Geometry check sheet. Reference: the model listing, model coordinates, mm. A direction names the side the tool comes from. Round coordinates to 2 decimals unless told otherwise and drop trailing zeros. Write each loop counter-clockwise with the first axis right and the second up, starting at its lowest first coordinate (ties: lowest second). Pieces come first, ordered by that corner, then holes. Notation, with made-up numbers: (-15, 0.5) - (-3, 0.5) arc R34 ccw to (-3, 35.5) - close; hole circle Ø7 at (15.5, 75). An arc over 180 degrees is marked (long way). Return JSON: item names as keys, results as strings. Group by question number.
from build123d import *

# Parameters (mm, degrees)
F1_DEPTH = 57.15
F2_R     = 3.175
F3_DEPTH = 50.801
F4_R     = 6.35
F5_DEPTH = 2.54
F6_R     = 2
F7_DEPTH = 50.801
F8_R     = 1.5875
F9_DEPTH = 12.7


with BuildPart() as f1:
    # F0 (on Front) → F1 (new body)
    with BuildSketch(Plane.XZ):
        Polygon((-25.4, 0), (0, 0), (25.4, 0), (25.4, 31.75), (18.796, 31.75), (18.796, 4.318), (0, 4.318), (-18.796, 4.318), (-18.796, 31.75), (-25.4, 31.75), align=None)
    extrude(amount=F1_DEPTH)

    # F2 (on face) → F3 (cut, through all)
    with BuildSketch(Plane(origin=(-25.4, 0, 0), x_dir=(0, -1, 0), z_dir=(-1, 0, 0))):
        with Locations((12.7, 12.7)):
            Circle(F2_R)
    extrude(amount=-F3_DEPTH, mode=Mode.SUBTRACT)

    # F4 (on face) → F5 (cut)
    with BuildSketch(Plane.XY.offset(4.318)):
        with Locations((0, -44.45)):
            Circle(F4_R)
    extrude(amount=-F5_DEPTH, mode=Mode.SUBTRACT)

    # F6 (on face) → F7 (cut, through all)
    with BuildSketch(Plane(origin=(-25.4, 0, 0), x_dir=(0, -1, 0), z_dir=(-1, 0, 0))):
        with Locations((38.1, 24.13)):
            Circle(F6_R)
        with Locations((47.6, 24.13)):
            Circle(F6_R)
    extrude(amount=-F7_DEPTH, mode=Mode.SUBTRACT)

    # F8 (on face) → F9 (cut)
    with BuildSketch(Plane.XY.offset(31.75)):
        with Locations((-22.098, -3.175)):
            Circle(F8_R)
        with Locations((-22.098, -22.225)):
            Circle(F8_R)
        with Locations((22.098, -3.175)):
            Circle(F8_R)
        with Locations((22.098, -22.225)):
            Circle(F8_R)
    extrude(amount=-F9_DEPTH, mode=Mode.SUBTRACT)


solid = f1.part
1. Material ranges on line 1 along X through (y, z) = (-22, 26.5); line 2 along X through (y, z) = (-55, 18); line 3 along Y through (x, z) = (-22, 24), recorded low to high.
2. Section check D-D (z = 24.13). State how many separate pieces and enclosed holes the cut face has, and give its area (3 significant figures).
3. Mould release check, pull along Y, two halves, no side actions. Record for faces 1 (the face through (0, -57.15, 4)), 2 (the face through (-22, -28, 31.75)), 3 (the face through (-22, -3, 19.05)): pulls with the +Y half, pulls with the -Y half, needs draft (parallel to the pull), parting line crosses it, or undercut.
4. Section check C-C (x = 0). Enter the section's corners in (y, z).
5. Section check A-A (y = -12.7). Enter the section's corners in (x, z) (3 decimals), and give its area (3 significant figures).
6. Section check B-B (z = 8). Enter the section's corners in (x, y).
7. Depth check by flat-ended pin: pin 1 Ø14 at (x, y) = (0, -45) entering from +Z; pin 2 Ø3.5 at (x, y) = (21.5, -3) entering from +Z; pin 3 Ø3 at (x, y) = (-22.098, -22.225) entering from +Z. Enter the tip coordinate at first touch or a pass-through.
8. Tool access check on faces 4 (the face through (22, -22, 19.05)), 5 (the face through (25.4, -28, 16)), 6 (the face through (0, -28, 4.318)). Record the directions out of +Z, -Z, +X, -X, +Y, -Y that give a thin tool (end or side, any length) a straight path to the whole face; none if there is none.
Result sheet:
{
 "1": {"line 1": "x = -25.4 to -23.67, -20.53 to -18.8, 18.8 to 20.53, 23.67 to 25.4", "line 2": "x = -25.4 to -18.8, 18.8 to 25.4", "line 3": "y = -57.15 to -49.6, -45.6 to -40.1, -36.1 to -23.81, -20.64 to -4.76, -1.59 to 0"},
 "2": {"separate pieces": "6", "enclosed holes": "4", "area": "618 mm²"},
 "3": {"face 1": "pulls with the -Y half", "face 2": "needs draft", "face 3": "undercut"},
 "4": {"outline": "(-57.15, 0) - (0, 0) - (0, 4.32) - (-38.1, 4.32) - (-38.1, 1.78) - (-50.8, 1.78) - (-50.8, 4.32) - (-57.15, 4.32) - close"},
 "5": {"outline": "(-25.4, 0) - (25.4, 0) - (25.4, 9.525) - (18.796, 9.525) - (18.796, 4.318) - (-18.796, 4.318) - (-18.796, 9.525) - (-25.4, 9.525) - close; (-25.4, 15.875) - (-18.796, 15.875) - (-18.796, 31.75) - (-25.4, 31.75) - close; (18.796, 15.875) - (25.4, 15.875) - (25.4, 31.75) - (18.796, 31.75) - close", "area": "498 mm²"},
 "6": {"outline": "(-25.4, -57.15) - (-18.8, -57.15) - (-18.8, 0) - (-25.4, 0) - close; (18.8, -57.15) - (25.4, -57.15) - (25.4, 0) - (18.8, 0) - close"},
 "7": {"pin 1": "stops at z = 4.32", "pin 2": "stops at z = 31.75", "pin 3": "stops at z = 19.05"},
 "8": {"face 4": "+Z", "face 5": "+Z, -Z, +X, +Y, -Y", "face 6": "+Z, +Y, -Y"}
}
